Autodesk Inventor part; units mm, degrees
ref_plane "YZ Plane" through (0, 0, 0) normal (1, 0, 0) x (0, 1, 0)
ref_plane "XZ Plane" through (0, 0, 0) normal (0, 1, 0) x (-1, 0, 0)
ref_plane "XY Plane" through (0, 0, 0) normal (0, 0, 1) x (1, 0, 0)
sketch "Sketch1" plane through (0, 0, 0) normal (0, 1, 0) x (-1, 0, 0)
  line L0 (11.5, 24) -> (-11.5, 24)
  line L1 (-11.5, 24) -> (-11.5, -24)
  line L2 (-11.5, -24) -> (11.5, -24)
  line L3 (11.5, -24) -> (11.5, 24)
  line L4 (11.5, 24) -> (-11.5, -24) construction
  line L5 (-11.5, 24) -> (11.5, -24) construction
  line L6 (-8.5, 21) -> (8.5, 21)
  line L7 (8.5, 21) -> (8.5, -21)
  line L8 (8.5, -21) -> (-8.5, -21)
  line L9 (-8.5, -21) -> (-8.5, 21)
  line L10 (-8.5, 21) -> (8.5, -21) construction
  line L11 (8.5, 21) -> (-8.5, -21) construction
  line L12 (0, 0) -> (-8.5, 0) construction
  circle A0 centre (0, -12) radius 1.5
  circle A1 centre (0, 12) radius 1.5
  line L13 (17.5, 30) -> (-17.5, 30)
  line L14 (-17.5, 30) -> (-17.5, -30)
  line L15 (-17.5, -30) -> (17.5, -30)
  line L16 (17.5, -30) -> (17.5, 30)
  line L17 (17.5, 30) -> (-17.5, -30) construction
  line L18 (-17.5, 30) -> (17.5, -30) construction
  circle A2 centre (14.5, 27) radius 1.5
  circle A3 centre (-14.5, 27) radius 1.5
  circle A4 centre (14.5, -27) radius 1.5
  circle A5 centre (-14.5, -27) radius 1.5
  dimension "d0" = 23
  dimension "d1" = 48
  dimension "d3" = 3
  dimension "d4" = 3
  dimension "d5" = 3
  dimension "d6" = 12
  dimension "d9" = 6
  dimension "d10" = 6
  dimension "d13" = 3
  dimension "d14" = 3
  dimension "d15" = 3
  dimension "d16" = 3
  dimension "d17" = 3
  dimension "d18" = 3
extrude "Extrusion1" add sketch "Sketch1" along normal blind 3 contours L16 L15 L14 L13
fillet "Fillet2" radius 1.5 8 edges at (17.5, 1.5, -30) (17.5, 1.5, 30) (-17.5, 1.5, 30) (-17.5, 1.5, -30) (11.5, 1.5, 24) (-11.5, 1.5, 24) (-11.5, 1.5, -24) (11.5, 1.5, -24)
sketch "Sketch2" plane through (0, 3, 0) normal (0, 1, 0) x (1, 0, 0)
  line L0 (-10, 24) -> (10, 24)
  line L1 (0, 24) -> (0, 29.9588) construction
  line L2 (0, 24) -> (-5, 24)
  line L3 (16, 30) -> (-16, 30)
  line L4 (-5, 24) -> (-10.0346, 30)
  line L5 (10, 24) -> (-10, 24)
  line L6 (-16, 30) -> (16, 30)
  line L7 (5, 24) -> (10.0346, 30)
  line L8 (-10.0346, 30) -> (10.0346, 30)
  point P0 (0, 0)
  dimension "d20" = 40
  dimension "d22" = 5
extrude "Extrusion2" cut sketch "Sketch2" against normal blind 10
properties part number "Middle external"
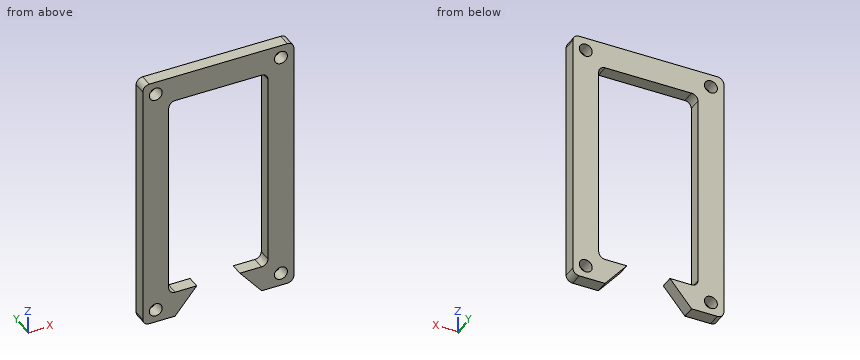
Model file for the job. Use its own axes, mm. Coordinates: 2 decimals unless noted, no trailing zeros. Order: outer loops, then holes, each group sorted by start corner. A loop starts at its lowest first (then second) coordinate and runs counter-clockwise, first axis right, second up. Notation, with made-up numbers: (31, 29) - (44, 29) arc R26 ccw to (44, 60) - close; hole circle Ø5 at (72, 22.25). An arc over 180 degrees is marked (long way). Return JSON: item names as keys, results as strings. Group by question number.
1) Saw through at C-C, the plane x = -14.5. Write the cut outline in (y, z).
2) Saw through at A-A, the plane z = -3.5. Write the cut outline in (x, y), plus the area to 3 significant figures.
3) Probe line 1 (Z direction, x = 14.5, y = 1.6); line 2 (X direction, y = 2.15, z = -6); line 3 (Z direction, x = 3, y = 0.7). List the from-to ranges inside material, lowest first. Write a range as from..to.
4) Saw through at B-B, the plane z = 27. Write the cut outline in (x, y), plus the area to 3 significant figures.
5) Saw through at D-D, the plane x = 9. Write the cut outline in (y, z), plus the area to 3 significant figures.
6) Flat gauge pin, fed straight in: P1, Ø1.5, axis at x = -3.5, y = 2, coming from the -Z side. Where does the tip first touch, or does it go through?
Values found:
{
 "1": {"outline": "(0, -30) - (3, -30) - (3, -28.5) - (0, -28.5) - close; (0, -25.5) - (3, -25.5) - (3, 25.5) - (0, 25.5) - close; (0, 28.5) - (3, 28.5) - (3, 30) - (0, 30) - close"},
 "2": {"outline": "(-17.5, 0) - (-11.5, 0) - (-11.5, 3) - (-17.5, 3) - close; (11.5, 0) - (17.5, 0) - (17.5, 3) - (11.5, 3) - close", "area": "36.0 mm²"},
 "3": {"line 1": "z = -30..-28.5, -25.5..25.5, 28.5..30", "line 2": "x = -17.5..-11.5, 11.5..17.5", "line 3": "z = 24..30"},
 "4": {"outline": "(-17.5, 0) - (-16, 0) - (-16, 3) - (-17.5, 3) - close; (-13, 0) - (13, 0) - (13, 3) - (-13, 3) - close; (16, 0) - (17.5, 0) - (17.5, 3) - (16, 3) - close", "area": "87.0 mm²"},
 "5": {"outline": "(0, -28.77) - (3, -28.77) - (3, -24) - (0, -24) - close; (0, 24) - (3, 24) - (3, 30) - (0, 30) - close", "area": "32.3 mm²"},
 "6": {"P1": "stops at z = 24"}
}
